CAD build for the part. Positions are in the model's coordinates, mm. A direction names the side the tool comes from. Give positions to 0.01 mm unless a question says otherwise; leave off trailing zeros. Write each loop counter-clockwise with the first axis right and the second up, starting at its lowest first coordinate (ties: lowest second). Pieces come first, ordered by that corner, then holes. Notation, with made-up numbers: (-29, -4.75) - (26, -4.75) arc R24 ccw to (26, 14.25) - close; hole circle Ø1 at (88, 72.5). An arc over 180 degrees is marked (long way). Answer as a JSON object with one key per item and string values.
from build123d import *

# Parameters (mm, degrees)
SKETCH1_W           = 63.5
SKETCH1_H           = 15.24
BOSS_EXTRUDE1_DEPTH = 7.62
BOSS_EXTRUDE2_DEPTH = 40.64
SKETCH3_R           = 5.715
BOSS_EXTRUDE3_DEPTH = 86.36
SKETCH4_R           = 1.905
CUT_EXTRUDE1_DEPTH  = 12.7


with BuildPart() as part:
    # Sketch1 → Boss-Extrude1 (new body)
    with BuildSketch(Plane(origin=(0, 0, 0), x_dir=(1, 0, 0), z_dir=(0, 1, 0))):
        with Locations((31.75, 7.62)):
            Rectangle(SKETCH1_W, SKETCH1_H)
    extrude(amount=BOSS_EXTRUDE1_DEPTH)

    # Sketch2 → Boss-Extrude2 (add)
    with BuildSketch(Plane.XY):
        with BuildLine():
            Line((-34.2099732, 38.1), (105.4900268, 38.1))
            ThreePointArc((105.4900268, 38.1), (120.7300268, 22.86), (105.4900268, 7.62))
            Line((105.4900268, 7.62), (-34.2099732, 7.62))
            ThreePointArc((-34.2099732, 7.62), (-49.4499732, 22.86), (-34.2099732, 38.1))
        make_face()
    extrude(amount=-BOSS_EXTRUDE2_DEPTH)

    # Sketch3 → Boss-Extrude3 (add)
    with BuildSketch(Plane.XZ):
        with Locations(Location((14.605, -7.62, 0), (0, 0, 270))):
            Circle(SKETCH3_R)
        with Locations(Location((48.895, -7.62, 0), (0, 0, 270))):
            Circle(SKETCH3_R)
    extrude(amount=BOSS_EXTRUDE3_DEPTH)

    # Sketch4 → Cut-Extrude1 (cut)
    with BuildSketch(Plane.XZ.offset(86.36)):
        with Locations(Location((14.605, -7.62, 0), (0, 0, 270))):
            Circle(SKETCH4_R)
        with Locations(Location((48.895, -7.62, 0), (0, 0, 270))):
            Circle(SKETCH4_R)
    extrude(amount=-CUT_EXTRUDE1_DEPTH, mode=Mode.SUBTRACT)


solid = part.part
(1) Saw through at A-A, the plane z = -7.62. Give the cut face in (x, y), and give its area (3 significant figures).
Answer key:
{"outline": "(-34.21, 7.62) - (0, 7.62) - (0, 0) - (8.89, 0) - (8.89, -86.36) - (12.7, -86.36) - (12.7, -73.66) - (16.51, -73.66) - (16.51, -86.36) - (20.32, -86.36) - (20.32, 0) - (43.18, 0) - (43.18, -86.36) - (46.99, -86.36) - (46.99, -73.66) - (50.8, -73.66) - (50.8, -86.36) - (54.61, -86.36) - (54.61, 0) - (63.5, 0) - (63.5, 7.62) - (105.49, 7.62) arc R15.24 ccw to (105.49, 38.1) - (-34.21, 38.1) arc R15.24 ccw to start", "area": "7,350 mm²"}
(2) Pull direction X, two halves, no side cores. Call faces 5 (the face through (35, 38.1, -20)), 6 (the face through (0, 4, -8)), 7 (the face through (43.825, -42.575, -10.257)): pulls with the +X half, pulls with the -X half, needs draft (parallel to the pull), parting line crosses it, or undercut.
Answer key:
{"face 5": "needs draft", "face 6": "pulls with the -X half", "face 7": "undercut"}
(3) Saw through at B-B, the plane x = 76.5. Give the cut face in (y, z).
Answer key:
{"outline": "(7.62, -40.64) - (38.1, -40.64) - (38.1, 0) - (7.62, 0) - close"}
(4) Saw through at D-D, the plane y = 3. Give the cut face in (x, z), and give its area (3 significant figures).
Answer key:
{"outline": "(0, -15.24) - (63.5, -15.24) - (63.5, 0) - (0, 0) - close", "area": "968 mm²"}
(5) Saw through at C-C, the plane y = -64. Give the cut face in (x, z) (3 decimals).
Answer key:
{"outline": "circle Ø11.43 at (14.605, -7.62); circle Ø11.43 at (48.895, -7.62)"}
(6) Probe L1, parallel to X at y = -79.25, z = -7.62; L2, parallel to X at y = -74, z = -8.5; L3, parallel to Y at x = 40, z = -13. List the from-to ranges inside material, lowest first. Write a range as [from, to].
Answer key:
{"L1": "x = [8.89, 12.7], [16.51, 20.32], [43.18, 46.99], [50.8, 54.61]", "L2": "x = [8.96, 12.92], [16.29, 20.25], [43.25, 47.21], [50.58, 54.54]", "L3": "y = [0, 38.1]"}
(7) 3-axis set-ups, long thin cutter, end or side, ignore diameter. For faces 1 (the face through (15, -73.66, -8)), 2 (the face through (63.5, 4, -8)), 3 (the face through (31, 4, -15.24)), 4 (the face through (37, 24, 0)): which of +Z, -Z, +X, -X, +Y, -Y reach the whole face in a straight line?
Answer key:
{"face 1": "-Y", "face 2": "+Z, -Z, +X, -Y", "face 3": "-Z, +X, -X, -Y", "face 4": "+Z, +X, -X, +Y, -Y"}
(8) Flat gauge pins, fed straight in: P1, Ø4, axis at x = 15, z = -8, coming from the -Y side; P2, Ø2, axis at y = -1.5, z = -9.5, coming from the -X side; P3, Ø6, axis at x = 43, y = -57, coming from the +Z side; P4, Ø1, axis at x = 41, z = -29, coming from the -Y side. Where does each tip first touch, or does it go through?
Answer key:
{"P1": "stops at y = -86.36", "P2": "stops at x = 8.96", "P3": "stops at z = -2.69", "P4": "stops at y = 7.62"}
